from build123d import *

# Parameters (mm, degrees)
F0_W     = 331.2
F0_H     = 207
F0_R     = 6
F1_DEPTH = 2
F2_R     = 2.5
F2_R_2   = 1.5
F3_DEPTH = 5
F5_DEPTH = 4


with BuildPart() as f1:
    # F0 (on Top) → F1 (new body)
    with BuildSketch(Plane.XY):
        with BuildLine():
            ThreePointArc((177.5, 129.5), (176.62132, 131.62132), (174.5, 132.5))
            Line((174.5, 132.5), (-174.5, 132.5))
            ThreePointArc((-174.5, 132.5), (-176.62132, 131.62132), (-177.5, 129.5))
            Line((-177.5, 129.5), (-177.5, -129.5))
            ThreePointArc((-177.5, -129.5), (-176.62132, -131.62132), (-174.5, -132.5))
            Line((-174.5, -132.5), (-147.5, -132.5))
            Line((-147.5, -132.5), (-147.5, -119.5))
            Line((-147.5, -119.5), (-102.5, -119.5))
            Line((-102.5, -119.5), (-102.5, -132.5))
            Line((-102.5, -132.5), (102.5, -132.5))
            Line((102.5, -132.5), (102.5, -119.5))
            Line((102.5, -119.5), (147.5, -119.5))
            Line((147.5, -119.5), (147.5, -132.5))
            Line((147.5, -132.5), (174.5, -132.5))
            ThreePointArc((174.5, -132.5), (176.62132, -131.62132), (177.5, -129.5))
            Line((177.5, -129.5), (177.5, 129.5))
        make_face()
        with Locations((0, 3)):
            Rectangle(F0_W, F0_H, mode=Mode.SUBTRACT)
        with Locations((0, 119.5)):
            Circle(F0_R, mode=Mode.SUBTRACT)
    extrude(amount=F1_DEPTH)

    # F2 (on face) → F3 (join)
    with BuildSketch(Plane(origin=(0, 0, 0), x_dir=(1, 0, 0), z_dir=(0, 0, -1))):
        with Locations((-169.5, 117.5)):
            Circle(F2_R)
        with Locations((-169.5, 117.5)):
            Circle(F2_R_2, mode=Mode.SUBTRACT)
        with Locations((168, 117.5)):
            Circle(F2_R)
        with Locations((168, 117.5)):
            Circle(F2_R_2, mode=Mode.SUBTRACT)
        with Locations((-169.5, -127.5)):
            Circle(F2_R)
        with Locations((-169.5, -127.5)):
            Circle(F2_R_2, mode=Mode.SUBTRACT)
        with Locations((168, -127.5)):
            Circle(F2_R)
        with Locations((168, -127.5)):
            Circle(F2_R_2, mode=Mode.SUBTRACT)
    extrude(amount=F3_DEPTH)

    # F4 (on face) → F5 (join)
    with BuildSketch(Plane(origin=(0, 0, 0), x_dir=(1, 0, 0), z_dir=(0, 0, -1))):
        with BuildLine():
            ThreePointArc((-177.5, -129.5), (-176.62132, -131.62132), (-174.5, -132.5))
            Line((-174.5, -132.5), (174.5, -132.5))
            ThreePointArc((174.5, -132.5), (176.62132, -131.62132), (177.5, -129.5))
            Line((177.5, -129.5), (177.5, 129.5))
            ThreePointArc((177.5, 129.5), (176.62132, 131.62132), (174.5, 132.5))
            Line((174.5, 132.5), (147.5, 132.5))
            Line((147.5, 132.5), (147.5, 119.5))
            Line((147.5, 119.5), (102.5, 119.5))
            Line((102.5, 119.5), (102.5, 132.5))
            Line((102.5, 132.5), (-102.5, 132.5))
            Line((-102.5, 132.5), (-102.5, 119.5))
            Line((-102.5, 119.5), (-147.5, 119.5))
            Line((-147.5, 119.5), (-147.5, 132.5))
            Line((-147.5, 132.5), (-174.5, 132.5))
            ThreePointArc((-174.5, 132.5), (-176.62132, 131.62132), (-177.5, 129.5))
            Line((-177.5, 129.5), (-177.5, -129.5))
        make_face()
        with BuildLine():
            ThreePointArc((-174.5, -131.5), (-175.914214, -130.914214), (-176.5, -129.5))
            Line((-176.5, -129.5), (-176.5, 129.5))
            ThreePointArc((-176.5, 129.5), (-175.914214, 130.914214), (-174.5, 131.5))
            Line((-174.5, 131.5), (-148.5, 131.5))
            Line((-148.5, 131.5), (-148.5, 118.5))
            Line((-148.5, 118.5), (-101.5, 118.5))
            Line((-101.5, 118.5), (-101.5, 131.5))
            Line((-101.5, 131.5), (101.5, 131.5))
            Line((101.5, 131.5), (101.5, 118.5))
            Line((101.5, 118.5), (148.5, 118.5))
            Line((148.5, 118.5), (148.5, 131.5))
            Line((148.5, 131.5), (174.5, 131.5))
            ThreePointArc((174.5, 131.5), (175.914214, 130.914214), (176.5, 129.5))
            Line((176.5, 129.5), (176.5, -129.5))
            ThreePointArc((176.5, -129.5), (175.914214, -130.914214), (174.5, -131.5))
            Line((174.5, -131.5), (-174.5, -131.5))
        make_face(mode=Mode.SUBTRACT)
    extrude(amount=F5_DEPTH)


solid = f1.part
Geometry check sheet. Reference: the model listing, model coordinates, mm. Coordinates: 2 decimals unless noted, no trailing zeros. Order: outer loops, then holes, each group sorted by start corner. A loop starts at its lowest first (then second) coordinate and runs counter-clockwise, first axis right, second up. Notation, with made-up numbers: (55.25, 26) -> (104.25, 26) arc R15 cw to (104.25, 34) -> close; hole circle Ø6 at (-0.75, 29). An arc over 180 degrees is marked (long way). Use a Markdown table: item, result. Add a question column.
1. Go/stop test with a flat-tipped pin: pin 1 Ø1.5 at (x, y) = (-169, -118) entering from -Z. Record where the tip stops, or that it passes through.
2. Mould release check, pull along X, two halves, no side actions. Record for faces 1 (the face through (-1, 109, 2)), 2 (the face through (-14, -107, 0)), 3 (the face through (-0.78, 125.45, 0.99)): pulls with the +X half, pulls with the -X half, needs draft (parallel to the pull), parting line crosses it, or undercut.
3. Cross-section at B-B (x = 153.5). Enter the section's corners in (y, z), and give its area (3 significant figures).
4. Cross-section at A-A (y = 119.5). Enter the section's corners in (x, z), and give its area (3 significant figures).
5. Cross-section at C-C (z = -2). Give the number of separate pieces and of enclosed holes in the cut face, and give its area (3 significant figures).
6. Cross-section at D-D (x = 0). Enter the section's corners in (y, z), and give its area (4 significant figures).
7. Material ranges on L1, parallel to Y at x = -169.5, z = -1.05; L2, parallel to X at y = -117.5, z = -2.05; L3, parallel to Y at x = 0, z = 1.1, recorded low to high.
Filled sheet:
| question | item | result |
|---|---|---|
| 1 | pin 1 | z = 0 |
| 2 | face 1 | needs draft |
| 2 | face 2 | undercut |
| 2 | face 3 | undercut |
| 3 | outline | (-132.5, -4) -> (-131.5, -4) -> (-131.5, 0) -> (-100.5, 0) -> (-100.5, 2) -> (-132.5, 2) -> close; (106.5, 0) -> (131.5, 0) -> (131.5, -4) -> (132.5, -4) -> (132.5, 2) -> (106.5, 2) -> close |
| 3 | area | 124 mm2 |
| 4 | outline | (-177.5, -4) -> (-176.5, -4) -> (-176.5, 0) -> (-6, 0) -> (-6, 2) -> (-177.5, 2) -> close; (6, 0) -> (176.5, 0) -> (176.5, -4) -> (177.5, -4) -> (177.5, 2) -> (6, 2) -> close |
| 4 | area | 694 mm2 |
| 5 | separate pieces | 5 |
| 5 | enclosed holes | 5 |
| 5 | area | 1,330 mm2 |
| 6 | outline | (-132.5, -4) -> (-131.5, -4) -> (-131.5, 0) -> (-100.5, 0) -> (-100.5, 2) -> (-132.5, 2) -> close; (106.5, 0) -> (113.5, 0) -> (113.5, 2) -> (106.5, 2) -> close; (125.5, 0) -> (131.5, 0) -> (131.5, -4) -> (132.5, -4) -> (132.5, 2) -> (125.5, 2) -> close |
| 6 | area | 100.0 mm2 |
| 7 | L1 | -132.5 to -131.5, -120 to -119, -116 to -115, 125 to 126, 129 to 130, 131.5 to 132.5 |
| 7 | L2 | -177.5 to -176.5, -172 to -171, -168 to -167, 165.5 to 166.5, 169.5 to 170.5, 176.5 to 177.5 |
| 7 | L3 | -132.5 to -100.5, 106.5 to 113.5, 125.5 to 132.5 |
